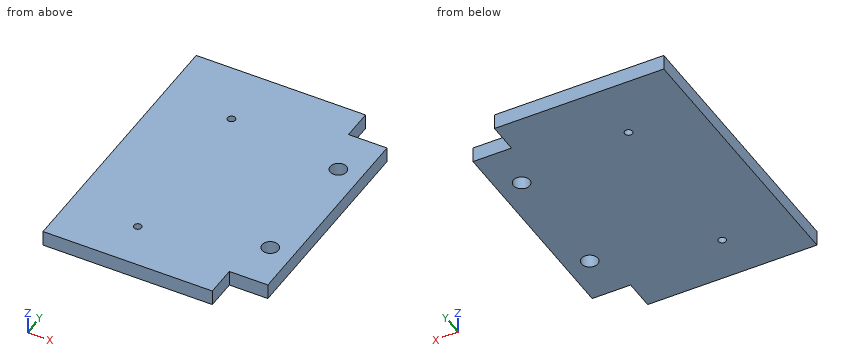
```python
from build123d import *

# Parameters (mm, degrees)
PAD_DEPTH       = 5
SKETCH001_R     = 1.25
POCKET_DEPTH    = 5
SKETCH002_R     = 2.65
POCKET001_DEPTH = 5


with BuildPart() as part:
    # Sketch → Pad (new body)
    with BuildSketch(Plane.XY):
        Polygon((-33.75, -45), (-33.75, 45), (21.25, 45), (21.25, 35), (33.75, 35), (33.75, -35), (21.25, -35), (21.25, -45), align=None)
    extrude(amount=PAD_DEPTH)

    # Sketch001 (on Face10 of Pad) → Pocket (cut)
    with BuildSketch(Plane.XY.offset(5)):
        with Locations((-11.25, 25)):
            Circle(SKETCH001_R)
        with Locations((-11.25, -30)):
            Circle(SKETCH001_R)
    extrude(amount=-POCKET_DEPTH, mode=Mode.SUBTRACT)

    # Sketch002 (on Face5 of Pocket) → Pocket001 (cut)
    with BuildSketch(Plane.XY.offset(5)):
        with Locations((26.25, 20)):
            Circle(SKETCH002_R)
        with Locations((26.25, -20)):
            Circle(SKETCH002_R)
    extrude(amount=-POCKET001_DEPTH, mode=Mode.SUBTRACT)


solid = part.part
```
Source: CAD feature listing. Evaluate the final solid. Frame: model axes, mm. Give positions to 0.01 mm unless a question says otherwise; leave off trailing zeros. Loops run counter-clockwise (first coordinate to the right, second up) from the corner with the lowest first, then second, coordinate; pieces in that order, holes last. Notation, with made-up numbers: (67, 2) -> (99, 2) arc R30 ccw to (99, 29) -> close; hole circle Ø9 at (-28.5, 57.5). An arc over 180 degrees is marked (long way). Put each result on its own line as item: value. Start each with the question number.
1) Cut plane B-B (y = 20). Return loops of the section in (x, z), then the cut area to 3 significant figures.
2) Cut plane D-D (y = -30). Return loops of the section in (x, z), then the cut area to 3 significant figures.
3) Contact query for a flat-ended pin moving along its axis: P1, Ø1.5, axis at y = 38.5, z = 2.5, coming from the +X side. Output: stop coordinate, or through.
4) Material intervals for probe 1 along Y at (x, z) = (26.25, 2.1); probe 2 along Y at (x, z) = (-11.25, 2.6); probe 3 along X at (y, z) = (22, 4.5), sorted ascending.
5) Cut plane C-C (x = -11.25). Return loops of the section in (y, z), then the cut area to 3 significant figures.
6) Cut plane A-A (z = 2.2). Return loops of the section in (x, y).
Results are:
1. outline: (-33.75, 0) -> (23.6, 0) -> (23.6, 5) -> (-33.75, 5) -> close; (28.9, 0) -> (33.75, 0) -> (33.75, 5) -> (28.9, 5) -> close
1. area: 311 mm2
2. outline: (-33.75, 0) -> (-12.5, 0) -> (-12.5, 5) -> (-33.75, 5) -> close; (-10, 0) -> (33.75, 0) -> (33.75, 5) -> (-10, 5) -> close
2. area: 325 mm2
3. P1: stops at x = 21.25
4. probe 1: y = -35 to -22.65, -17.35 to 17.35, 22.65 to 35
4. probe 2: y = -45 to -31.25, -28.75 to 23.75, 26.25 to 45
4. probe 3: x = -33.75 to 24.51, 27.99 to 33.75
5. outline: (-45, 0) -> (-31.25, 0) -> (-31.25, 5) -> (-45, 5) -> close; (-28.75, 0) -> (23.75, 0) -> (23.75, 5) -> (-28.75, 5) -> close; (26.25, 0) -> (45, 0) -> (45, 5) -> (26.25, 5) -> close
5. area: 425 mm2
6. outline: (-33.75, -45) -> (21.25, -45) -> (21.25, -35) -> (33.75, -35) -> (33.75, 35) -> (21.25, 35) -> (21.25, 45) -> (-33.75, 45) -> close; hole circle Ø2.5 at (-11.25, -30); hole circle Ø2.5 at (-11.25, 25); hole circle Ø5.3 at (26.25, -20); hole circle Ø5.3 at (26.25, 20)
